Geometry: final body of the model. Coordinates: model frame, mm. A direction names the side the tool comes from. Coordinates: 2 decimals unless noted, no trailing zeros. Loops run counter-clockwise (first coordinate to the right, second up) from the corner with the lowest first, then second, coordinate; pieces in that order, holes last. Notation, with made-up numbers: (9, -15) -> (41, -15) arc R14 ccw to (41, -5) -> close; hole circle Ø9 at (86.5, -24). An arc over 180 degrees is marked (long way). One line per item, written item: value. Start each with the question number.
from build123d import *

# Parameters (mm, degrees)
BUITENAFMETING_RECHTHOEK_W  = 90
BUITENAFMETING_RECHTHOEK_H  = 40
PLAAT_DEPTH                 = 4
TAND_HOR_W                  = 12.857142857
TAND_HOR_H                  = 4
TAND_BOVEN_DEPTH            = 5
TANDEN_PATROON_BOVEN_COUNT  = 4
TANDEN_PATROON_BOVEN_PITCH  = 25.714285714
TAND_VER_W                  = 4
TAND_VER_H                  = 8
TAND_LINKS_DEPTH            = 5
TANDEN_PATROON_LINKS_COUNT  = 2
TANDEN_PATROON_LINKS_PITCH  = 16
TAND_O_W                    = 12.857142857
TAND_O_H                    = 4
TAND_ONDER_DEPTH            = 5
TANDEN_PATROON_ONDER_COUNT  = 4
TANDEN_PATROON_ONDER_PITCH  = 25.714285714
TAND_R_W                    = 4
TAND_R_H                    = 8
TAND_RECHTS_DEPTH           = 5
TANDEN_PATROON_RECHTS_COUNT = 2
TANDEN_PATROON_RECHTS_PITCH = 16


with BuildPart() as part:
    # Buitenafmeting Rechthoek → Plaat (new body)
    with BuildSketch(Plane.XY):
        with Locations((45, 20)):
            Rectangle(BUITENAFMETING_RECHTHOEK_W, BUITENAFMETING_RECHTHOEK_H)
    extrude(amount=-PLAAT_DEPTH)

    # Tand Hor → Tand Boven (cut, through all)
    with BuildSketch(Plane.XY):
        with Locations((6.428571429, 38)):
            Rectangle(TAND_HOR_W, TAND_HOR_H)
    tand_boven = extrude(amount=-TAND_BOVEN_DEPTH, mode=Mode.SUBTRACT)

    # Tanden Patroon Boven: Tand Boven ×4
    with Locations(*[(i * TANDEN_PATROON_BOVEN_PITCH, 0, 0) for i in range(1, TANDEN_PATROON_BOVEN_COUNT)]):
        add(tand_boven, mode=Mode.SUBTRACT)

    # Tand Ver → Tand Links (cut, through all)
    with BuildSketch(Plane.XY):
        with Locations((2, 28)):
            Rectangle(TAND_VER_W, TAND_VER_H)
    tand_links = extrude(amount=-TAND_LINKS_DEPTH, mode=Mode.SUBTRACT)

    # Tanden Patroon Links: Tand Links ×2
    with Locations(*[(0, -i * TANDEN_PATROON_LINKS_PITCH, 0) for i in range(1, TANDEN_PATROON_LINKS_COUNT)]):
        add(tand_links, mode=Mode.SUBTRACT)

    # Tand O → Tand Onder (cut, through all)
    with BuildSketch(Plane.XY):
        with Locations((6.428571429, 2)):
            Rectangle(TAND_O_W, TAND_O_H)
    tand_onder = extrude(amount=-TAND_ONDER_DEPTH, mode=Mode.SUBTRACT)

    # Tanden Patroon Onder: Tand Onder ×4
    with Locations(*[(i * TANDEN_PATROON_ONDER_PITCH, 0, 0) for i in range(1, TANDEN_PATROON_ONDER_COUNT)]):
        add(tand_onder, mode=Mode.SUBTRACT)

    # Tand R → Tand Rechts (cut, through all)
    with BuildSketch(Plane.XY):
        with Locations((88, 28)):
            Rectangle(TAND_R_W, TAND_R_H)
    tand_rechts = extrude(amount=-TAND_RECHTS_DEPTH, mode=Mode.SUBTRACT)

    # Tanden Patroon Rechts: Tand Rechts ×2
    with Locations(*[(0, -i * TANDEN_PATROON_RECHTS_PITCH, 0) for i in range(1, TANDEN_PATROON_RECHTS_COUNT)]):
        add(tand_rechts, mode=Mode.SUBTRACT)


solid = part.part
1. Line query: L1, parallel to X at y = 38.5, z = -2.2; L2, parallel to Y at x = 83, z = -3.6; L3, parallel to X at y = 13, z = -1.7. Output: solid intervals per line, ascending. Write a range as [from, to].
2. Section C-C on y = 30.5. Return the cut outline in (x, z), plus the area to 3 significant figures.
3. Draft query along X for faces 1 (the face through (64.286, 38, -2)), 2 (the face through (2, 8, -2)), 3 (the face through (0, 6, -2)). Return one class per face: released by +X, released by -X, zero draft, split by the parting line, or undercut.
4. Section A-A on y = 37. Return the cut outline in (x, z).
5. Set-up query: faces 4 (the face through (12.857, 2, -2)), 5 (the face through (83, 36, -2)), 6 (the face through (12.857, 38, -2)), 7 (the face through (51.429, 38, -2)). Return all of +Z, -Z, +X, -X, +Y, -Y with unobstructed straight access to the full face (end or side cutting, diameter ignored); none if empty.
6. Pin query (flat end, axial travel): pin 1 Ø1.2 at (x, z) = (2, -1) entering from +Y; pin 2 Ø2 at (y, z) = (1.5, -2.5) entering from -X; pin 3 Ø1.2 at (y, z) = (11, -2) entering from +X. Return the tip coordinate at first contact, or that it passes through.
7. Section B-B on x = 83.5. Return the cut outline in (y, z), plus the area to 3 significant figures.
Checks:
1. L1: [12.86, 25.71], [38.57, 51.43], [64.29, 77.14]
1. L2: [4, 36]
1. L3: [4, 86]
2. outline: (4, -4) -> (86, -4) -> (86, 0) -> (4, 0) -> close
2. area: 328 mm²
3. face 1: undercut
3. face 2: zero draft
3. face 3: released by -X
4. outline: (12.86, -4) -> (25.71, -4) -> (25.71, 0) -> (12.86, 0) -> close; (38.57, -4) -> (51.43, -4) -> (51.43, 0) -> (38.57, 0) -> close; (64.29, -4) -> (77.14, -4) -> (77.14, 0) -> (64.29, 0) -> close
5. face 4: +Z, -Z, -X, -Y
5. face 5: +Z, -Z, +X, +Y
5. face 6: +Z, -Z, -X, +Y
5. face 7: +Z, -Z, +Y
6. pin 1: y = 36
6. pin 2: x = 12.86
6. pin 3: x = 86
7. outline: (4, -4) -> (36, -4) -> (36, 0) -> (4, 0) -> close
7. area: 128 mm²
